```python
from build123d import *

# Parameters (mm, degrees)
F0_W      = 50
F0_H      = 50
F1_DEPTH  = 50
F2_W      = 20
F2_H      = 20
F3_DEPTH  = 25
F4_R      = 4
F5_DEPTH  = 40
F6_R      = 4
F7_DEPTH  = 40
F8_R      = 4
F10_DEPTH = 60
F9_R      = 3.879999
F11_DEPTH = 60
F12_R     = 10
F13_R     = 10
F14_R     = 10
F15_R     = 10
F16_R     = 3
F17_R     = 5


with BuildPart() as f1:
    # F0 (on Top) → F1 (new body)
    with BuildSketch(Plane.XY):
        with Locations((25, 25)):
            Rectangle(F0_W, F0_H)
    extrude(amount=F1_DEPTH)

    # F2 (on face) → F3 (join)
    with BuildSketch(Plane.XY.offset(50)):
        with Locations((25, 24.755215)):
            Rectangle(F2_W, F2_H)
    extrude(amount=F3_DEPTH)

    # F4 (on face) → F5 (join)
    with BuildSketch(Plane.YZ.offset(50)):
        with Locations((26, 24)):
            Circle(F4_R)
    extrude(amount=F5_DEPTH)

    # F6 (on face) → F7 (join)
    with BuildSketch(Plane(origin=(0, 0, 0), x_dir=(0, -1, 0), z_dir=(-1, 0, 0))):
        with Locations((-24, 24)):
            Circle(F6_R)
    extrude(amount=F7_DEPTH)

    # F8 (on face) → F10 (join)
    with BuildSketch(Plane(origin=(0, 0, 0), x_dir=(1, 0, 0), z_dir=(0, 0, -1))):
        with Locations((14, -26.046494)):
            Circle(F8_R)
    extrude(amount=F10_DEPTH)

    # F9 (on face) → F11 (join)
    with BuildSketch(Plane(origin=(0, 0, 0), x_dir=(1, 0, 0), z_dir=(0, 0, -1))):
        with Locations((36.120001, -26.120001)):
            Circle(F9_R)
    extrude(amount=F11_DEPTH)

    # F12
    f12_edges = [f1.edges().sort_by_distance(p)[0] for p in [
        (25, 0, 50),
    ]]
    fillet(f12_edges, radius=F12_R)

    # F13
    f13_edges = [f1.edges().sort_by_distance(p)[0] for p in [
        (25, 50, 50),
    ]]
    fillet(f13_edges, radius=F13_R)

    # F14
    f14_edges = [f1.edges().sort_by_distance(p)[0] for p in [
        (50, 25, 50),
    ]]
    fillet(f14_edges, radius=F14_R)

    # F15
    f15_edges = [f1.edges().sort_by_distance(p)[0] for p in [
        (0, 25, 50),
    ]]
    fillet(f15_edges, radius=F15_R)

    # F16
    f16_edges = [f1.edges().sort_by_distance(p)[0] for p in [
        (25, 34.755215, 75),
        (15, 34.755215, 62.5),
        (35, 34.755215, 62.5),
        (15, 24.755215, 75),
        (15, 14.755215, 62.5),
        (25, 14.755215, 75),
        (35, 14.755215, 62.5),
        (35, 24.755215, 75),
    ]]
    fillet(f16_edges, radius=F16_R)

    # F17
    f17_edges = [f1.edges().sort_by_distance(p)[0] for p in [
        (25, 0, 0),
    ]]
    fillet(f17_edges, radius=F17_R)


solid = f1.part
```
The listing builds one solid part. Answer for the finished solid, in the listing's coordinates (mm). A direction names the side the tool comes from. Coordinates: 2 decimals unless noted, no trailing zeros. Loops run counter-clockwise (first coordinate to the right, second up) from the corner with the lowest first, then second, coordinate; pieces in that order, holes last. Notation, with made-up numbers: (77.25, 74) - (107.25, 74) arc R28 cw to (107.25, 104) - close; hole circle Ø11 at (-10, 44). An arc over 180 degrees is marked (long way). Use a Markdown table: item, result. Add a question column.
1) Find the intervals of material crossed by line 1 (Z direction, x = -27, y = 24); line 2 (Z direction, x = 22.5, y = 29); line 3 (X direction, y = 19.5, z = 21.5), in increasing order.
2) The part is cut by section B-B, the plane z = 24. Give the vertices of the cut face in (x, y), and give its area (3 significant figures).
3) The part is cut by section D-D, the plane x = -11.5. Give the vertices of the cut face in (y, z).
4) Given pin 1 (11 mm diameter, centred on x = 23.5, z = 59, fed in from -Y); pin 2 (15.5 mm diameter, centred on y = 21.5, z = 61, fed in from -X); pin 3 (1.5 mm diameter, centred on x = 46, y = 32, fed in from -Z), each flat-ended and moving along its own axis, determine where each tip first touches the part or whether it passes through.
5) The part is cut by section A-A, the plane y = 12. Give the vertices of the cut face in (x, z), and give its area (3 significant figures).
6) For faces 1 (the flat face through (25, 35, 50)), 2 (the flat face through (25, 14.755, 61)), 3 (the cylindrical face through (15.9, 33.9, 61.2)), 4 (the flat face through (25, 34.755, 61)), 5 (the cylindrical face through (69.72, 25.479, 27.966)), determine the directions among +Z, -Z, +X, -X, +Y, -Y from which every point of the face is accessible in a straight line to the end or side of a thin tool.
7) The part is cut by section C-C, the plane z = 57. Give the vertices of the cut face in (x, y).
Here are the results:
| question | item | result |
|---|---|---|
| 1 | line 1 | z = 20 to 28 |
| 1 | line 2 | z = 0 to 75 |
| 1 | line 3 | x = 0 to 50 |
| 2 | outline | (-40, 20) - (0, 20) - (0, 10) arc R10 ccw to (10, 0) - (40, 0) arc R10 ccw to (50, 10) - (50, 22) - (90, 22) - (90, 30) - (50, 30) - (50, 40) arc R10 ccw to (40, 50) - (10, 50) arc R10 ccw to (0, 40) - (0, 28) - (-40, 28) - close |
| 2 | area | 3,050 mm^2 |
| 3 | outline | circle Ø8 at (24, 24) |
| 4 | pin 1 | stops at y = 14.76 |
| 4 | pin 2 | stops at x = 15 |
| 4 | pin 3 | stops at z = 0.01 |
| 5 | outline | (0, 5) arc R5 ccw to (5, 0) - (45, 0) arc R5 ccw to (50, 5) - (50, 40) arc R10 ccw to (40, 50) - (10, 50) arc R10 ccw to (0, 40) - close |
| 5 | area | 2,450 mm^2 |
| 6 | face 1 | +Z |
| 6 | face 2 | +Z, +X, -X, -Y |
| 6 | face 3 | +Z, -X, +Y |
| 6 | face 4 | +Z, +X, -X, +Y |
| 6 | face 5 | +X |
| 7 | outline | (15, 17.76) arc R3 ccw to (18, 14.76) - (32, 14.76) arc R3 ccw to (35, 17.76) - (35, 31.76) arc R3 ccw to (32, 34.76) - (18, 34.76) arc R3 ccw to (15, 31.76) - close |
